Here's how the part is built. I have some questions about the finished solid (model axes, mm). Give positions to 0.01 mm unless a question says otherwise; leave off trailing zeros. Order: outer loops, then holes, each group sorted by start corner. A loop starts at its lowest first (then second) coordinate and runs counter-clockwise, first axis right, second up. Notation, with made-up numbers: (-11, -4.5) - (-6, -4.5) arc R36 cw to (-6, 30.5) - close; hole circle Ø9 at (1.25, 31.5). An arc over 180 degrees is marked (long way). One line per question, with ' | ' between items.
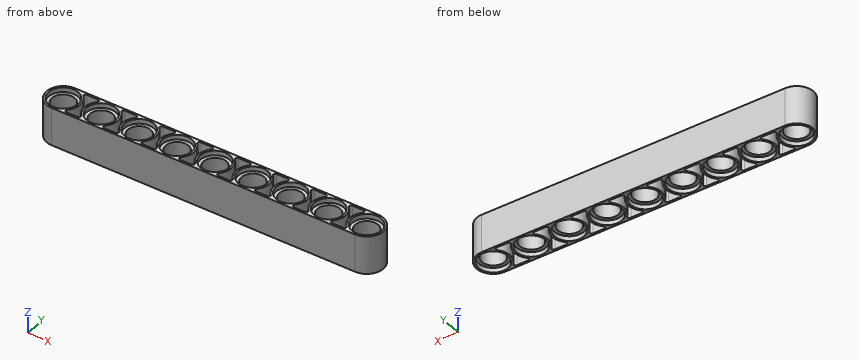
from build123d import *

# Parameters (mm, degrees)
BOSS_EXTRUDE2_DEPTH = 8
SKETCH5_R           = 3.1
CUT_EXTRUDE4_DEPTH  = 1
CUT_EXTRUDE5_START  = -1
SKETCH6_R           = 3.1
CUT_EXTRUDE5_DEPTH  = 1
SKETCH7_R           = 2.4
CUT_EXTRUDE6_DEPTH  = 68.952189074
LPATTERN1_COUNT     = 9
LPATTERN1_PITCH     = 8
CUT_EXTRUDE7_DEPTH  = 69.062471304
LPATTERN2_COUNT     = 8
LPATTERN2_PITCH     = 8


with BuildPart() as part:
    # Sketch1 → Boss-Extrude2 (new body)
    with BuildSketch(Plane.XY):
        with BuildLine():
            Line((0, -3.5), (-64, -3.5))
            ThreePointArc((-64, -3.5), (-67.5, 0), (-64, 3.5))
            Line((-64, 3.5), (0, 3.5))
            ThreePointArc((0, 3.5), (3.5, 0), (0, -3.5))
        make_face()
    extrude(amount=BOSS_EXTRUDE2_DEPTH)

    # Sketch5 → Cut-Extrude4 (cut)
    with BuildSketch(Plane(origin=(0, 0, 0), x_dir=(-1, 0, 0), z_dir=(0, 0, -1))):
        Circle(SKETCH5_R)
    cut_extrude4 = extrude(amount=-CUT_EXTRUDE4_DEPTH, mode=Mode.SUBTRACT)

    # Sketch6 → Cut-Extrude5 (cut)
    with BuildSketch(Plane.XY.offset(8).offset(CUT_EXTRUDE5_START)):
        with Locations(Location((0, 0, 0), (0, 0, 180))):
            Circle(SKETCH6_R)
    cut_extrude5 = extrude(amount=CUT_EXTRUDE5_DEPTH, mode=Mode.SUBTRACT)

    # Sketch7 → Cut-Extrude6 (cut, symmetric)
    with BuildSketch(Plane.XY.offset(7)):
        Circle(SKETCH7_R)
    cut_extrude6 = extrude(amount=CUT_EXTRUDE6_DEPTH, both=True, mode=Mode.SUBTRACT)

    # LPattern1: Cut-Extrude4, Cut-Extrude5, Cut-Extrude6 ×9
    with Locations(*[(-i * LPATTERN1_PITCH, 0, 0) for i in range(1, LPATTERN1_COUNT)]):
        add(cut_extrude4, mode=Mode.SUBTRACT)
        add(cut_extrude5, mode=Mode.SUBTRACT)
        add(cut_extrude6, mode=Mode.SUBTRACT)

    # Sketch8 → Cut-Extrude7 (cut, through all)
    with BuildSketch(Plane(origin=(0, 0, 0), x_dir=(-1, 0, 0), z_dir=(0, 0, -1))):
        with BuildLine():
            Line((2.814249456, 3.1), (5.185750544, 3.1))
            ThreePointArc((5.185750544, 3.1), (5.553697029, 2.856892908), (5.474391514, 2.423076923))
            ThreePointArc((5.474391514, 2.423076923), (4.5, 0), (5.474391514, -2.423076923))
            ThreePointArc((5.474391514, -2.423076923), (5.553697029, -2.856892908), (5.185750544, -3.1))
            Line((5.185750544, -3.1), (2.814249456, -3.1))
            ThreePointArc((2.814249456, -3.1), (2.446302971, -2.856892908), (2.525608486, -2.423076923))
            ThreePointArc((2.525608486, -2.423076923), (3.5, 0), (2.525608486, 2.423076923))
            ThreePointArc((2.525608486, 2.423076923), (2.446302971, 2.856892908), (2.814249456, 3.1))
        make_face()
    cut_extrude7 = extrude(amount=-CUT_EXTRUDE7_DEPTH, mode=Mode.SUBTRACT)

    # LPattern2: Cut-Extrude7 ×8
    with Locations(*[(-i * LPATTERN2_PITCH, 0, 0) for i in range(1, LPATTERN2_COUNT)]):
        add(cut_extrude7, mode=Mode.SUBTRACT)


solid = part.part
1) I'm going to push flat-ended pins straight in: P1, Ø3, axis at x = -15, y = 0.5, coming from the +Z side; P2, Ø1.5, axis at y = -2.5, z = 5, coming from the -X side; P3, Ø4, axis at y = 1.5, z = 4, coming from the +X side. Where does each tip first touch, or does it pass through?
Model answer:
P1: stops at z = 7 | P2: stops at x = -67.03 | P3: stops at x = 3.5
2) I want a section at B-B (y = 0). State how many separate pieces and enclosed holes the cut face has, plus the area to 3 significant figures.
Model answer:
separate pieces: 18 | enclosed holes: 0 | area: 133 mm2
3) I want a section at A-A (x = -8). List the corners of the cut face in (y, z) for me.
Model answer:
outline: (-3.5, 0) - (-3.1, 0) - (-3.1, 1) - (-2.4, 1) - (-2.4, 7) - (-3.1, 7) - (-3.1, 8) - (-3.5, 8) - close; (2.4, 1) - (3.1, 1) - (3.1, 0) - (3.5, 0) - (3.5, 8) - (3.1, 8) - (3.1, 7) - (2.4, 7) - close
4) Please list where these lines run through material, in increasing order: L1, parallel to Y at x = -24, z = 3.25; L2, parallel to Y at x = -48, z = 7.3; L3, parallel to Y at x = -53, z = 4.25.
Model answer:
L1: y = -3.5 to -2.4, 2.4 to 3.5 | L2: y = -3.5 to -3.1, 3.1 to 3.5 | L3: y = -3.5 to -3.1, -1.8 to 1.8, 3.1 to 3.5
5) I want a section at D-D (x = -32.5). List the corners of the cut face in (y, z) for me, plus the area to 3 significant figures.
Model answer:
outline: (-3.5, 0) - (-3.06, 0) - (-3.06, 1) - (-2.35, 1) - (-2.35, 7) - (-3.06, 7) - (-3.06, 8) - (-3.5, 8) - close; (2.35, 1) - (3.06, 1) - (3.06, 0) - (3.5, 0) - (3.5, 8) - (3.06, 8) - (3.06, 7) - (2.35, 7) - close | area: 15.6 mm2
